Read the model definition and answer for the solid it produces. Units are mm, in the model's axes. Give positions to 0.01 mm unless a question says otherwise; leave off trailing zeros. Loops run counter-clockwise (first coordinate to the right, second up) from the corner with the lowest first, then second, coordinate; pieces in that order, holes last. Notation, with made-up numbers: (24, 26.25) -> (32, 26.25) arc R14 ccw to (32, 34.25) -> close; hole circle Ø8 at (-26.75, 31). An arc over 180 degrees is marked (long way). Return JSON: item names as keys, results as strings. Group by question number.
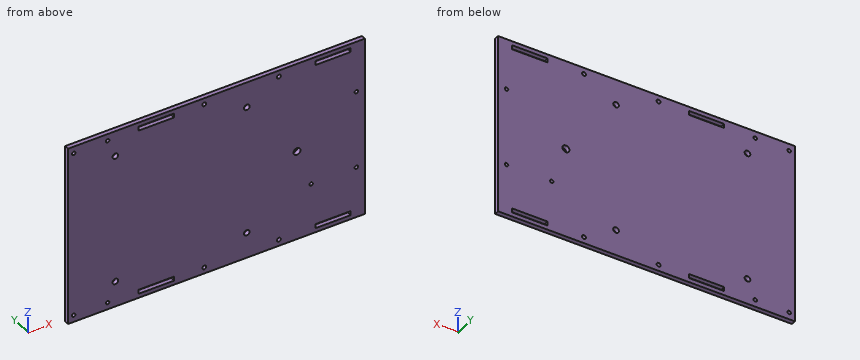
from build123d import *

# Parameters (mm, degrees)
SKETCH2_W         = 210
SKETCH2_H         = 130
SKETCH2_R         = 2
SKETCH2_R_2       = 1.25
MAIN_DEPTH        = 3.2
SKETCH3_R         = 1.25
MOTOR_MOUNT_DEPTH = 3.2
SKETCH4_R         = 1.4
SKETCH4_W         = 25
SKETCH4_H         = 3
SIDE_HOLES_DEPTH  = 3.2
SKETCH5_R         = 2.5
BACK_WHEEL_DEPTH  = 3.2


with BuildPart() as part:
    # Sketch2 → main (new body)
    with BuildSketch(Plane(origin=(0, 0, 0), x_dir=(1, 0, 0), z_dir=(0, 1, 0))):
        with Locations((25, 0)):
            Rectangle(SKETCH2_W, SKETCH2_H)
        with Locations(Location((-46.5, 46.5, 0), (0, 0, 270))):
            Circle(SKETCH2_R, mode=Mode.SUBTRACT)
        with Locations(Location((46.5, 46.5, 0), (0, 0, 270))):
            Circle(SKETCH2_R, mode=Mode.SUBTRACT)
        with Locations(Location((-46.5, -46.5, 0), (0, 0, 270))):
            Circle(SKETCH2_R, mode=Mode.SUBTRACT)
        with Locations(Location((46.5, -46.5, 0), (0, 0, 270))):
            Circle(SKETCH2_R, mode=Mode.SUBTRACT)
        with Locations(Location((92, 28, 0), (0, 0, 270))):
            Circle(SKETCH2_R_2, mode=Mode.SUBTRACT)
        with Locations(Location((124, 28, 0), (0, 0, 270))):
            Circle(SKETCH2_R_2, mode=Mode.SUBTRACT)
        with Locations(Location((124, -28, 0), (0, 0, 270))):
            Circle(SKETCH2_R_2, mode=Mode.SUBTRACT)
    extrude(amount=MAIN_DEPTH)

    # Sketch3 → motor mount (cut)
    with BuildSketch(Plane(origin=(0, 3.2, 0), x_dir=(1, 0, 0), z_dir=(0, 1, 0))):
        with Locations(Location((-76, -60, 0), (0, 0, 270))):
            Circle(SKETCH3_R)
        with Locations(Location((-52, -60, 0), (0, 0, 270))):
            Circle(SKETCH3_R)
        with Locations(Location((-52, 60, 0), (0, 0, 270))):
            Circle(SKETCH3_R)
        with Locations(Location((-76, 60, 0), (0, 0, 270))):
            Circle(SKETCH3_R)
    extrude(amount=-MOTOR_MOUNT_DEPTH, mode=Mode.SUBTRACT)

    # Sketch4 → side holes (cut)
    with BuildSketch(Plane(origin=(0, 3.2, 0), x_dir=(1, 0, 0), z_dir=(0, 1, 0))):
        with Locations(Location((16.4, -60.5, 0), (0, 0, 270))):
            Circle(SKETCH4_R)
        with Locations(Location((69.2, -60.5, 0), (0, 0, 270))):
            Circle(SKETCH4_R)
        with Locations(Location((69.2, 60.5, 0), (0, 0, 270))):
            Circle(SKETCH4_R)
        with Locations(Location((16.4, 60.5, 0), (0, 0, 270))):
            Circle(SKETCH4_R)
        with Locations((-17.5, -60.5)):
            Rectangle(SKETCH4_W, SKETCH4_H)
        with Locations((107.5, -60.5)):
            Rectangle(SKETCH4_W, SKETCH4_H)
        with Locations((107.5, 60.5)):
            Rectangle(SKETCH4_W, SKETCH4_H)
        with Locations((-17.5, 60.5)):
            Rectangle(SKETCH4_W, SKETCH4_H)
    extrude(amount=-SIDE_HOLES_DEPTH, mode=Mode.SUBTRACT)

    # Sketch5 → back wheel (cut)
    with BuildSketch(Plane(origin=(0, 3.2, 0), x_dir=(1, 0, 0), z_dir=(0, 1, 0))):
        with Locations(Location((82, 0, 0), (0, 0, 270))):
            Circle(SKETCH5_R)
    extrude(amount=-BACK_WHEEL_DEPTH, mode=Mode.SUBTRACT)


solid = part.part
1. Straight lines are drawn through the part: line 1 (Z direction, x = 124, y = 1.15); line 2 (Z direction, x = -17, y = 0.45); line 3 (X direction, y = 2.3, z = -46.5). For each, find the intervals that lie inside material, in ascending order. Write a range as from..to.
2. Section C-C on z = 46.5 is taken. Determine the outline of the cut face in (x, y).
3. Section D-D on y = 2.7 is taken. State how many separate pieces and enclosed holes the cut face has, then the cut area to 3 significant figures.
4. Section B-B on x = 82 is taken. Determine the outline of the cut face in (y, z), then the cut area to 3 significant figures.
5. Section A-A on z = 0 is taken. Determine the outline of the cut face in (x, y), then the cut area to 3 significant figures.
Completed:
{
 "1": {"line 1": "z = -65..-29.25, -26.75..26.75, 29.25..65", "line 2": "z = -65..-62, -59..59, 62..65", "line 3": "x = -80..-48.5, -44.5..44.5, 48.5..130"},
 "2": {"outline": "(-80, 0) -> (-48.5, 0) -> (-48.5, 3.2) -> (-80, 3.2) -> close; (-44.5, 0) -> (44.5, 0) -> (44.5, 3.2) -> (-44.5, 3.2) -> close; (48.5, 0) -> (130, 0) -> (130, 3.2) -> (48.5, 3.2) -> close"},
 "3": {"separate pieces": "1", "enclosed holes": "20", "area": "26,900 mm²"},
 "4": {"outline": "(0, -65) -> (3.2, -65) -> (3.2, -2.5) -> (0, -2.5) -> close; (0, 2.5) -> (3.2, 2.5) -> (3.2, 65) -> (0, 65) -> close", "area": "400 mm²"},
 "5": {"outline": "(-80, 0) -> (79.5, 0) -> (79.5, 3.2) -> (-80, 3.2) -> close; (84.5, 0) -> (130, 0) -> (130, 3.2) -> (84.5, 3.2) -> close", "area": "656 mm²"}
}
